Autodesk Inventor part; units mm, degrees
ref_plane "YZ Plane" through (0, 0, 0) normal (1, 0, 0) x (0, 1, 0)
ref_plane "XZ Plane" through (0, 0, 0) normal (0, 1, 0) x (-1, 0, 0)
ref_plane "XY Plane" through (0, 0, 0) normal (0, 0, 1) x (1, 0, 0)
sketch "Sketch1" plane through (0, 0, 0) normal (0, 1, 0) x (-1, 0, 0)
  line L0 (22.75, -10.36) -> (7.75, -10.36)
  line L1 (7.75, -10.36) -> (-0.1031, 0)
  circle A0 centre (4.34, -10.36) radius 1
  line L2 (22.75, 10.36) -> (7.75, 10.36)
  circle A1 centre (12.64, 0) radius 9.6 construction
  line L3 (22.75, 12.36) -> (22.75, -12.36)
  circle A2 centre (4.34, 10.36) radius 1
  line L4 (7.75, 10.36) -> (-0.1031, 0)
  line L5 (26.25, 19) -> (26.25, -19)
  line L6 (22.75, -12.36) -> (-22.75, -12.36)
  line L7 (22.75, 0) -> (-22.75, 0) construction
  line L8 (26.25, -19) -> (-28.75, -19)
  line L9 (26.25, -19) -> (-28.75, 19) construction
  line L10 (-28.75, -19) -> (26.25, 19) construction
  line L11 (-22.75, 12.36) -> (22.75, 12.36)
  line L12 (-28.75, 19) -> (26.25, 19)
  line L13 (-28.75, -19) -> (-28.75, 19)
  circle A3 centre (-16.36, 10.25) radius 1
  line L14 (-22.75, -12.36) -> (-22.75, 12.36)
  circle A4 centre (-16.36, -10.25) radius 1
  point P0 (0, 0)
  point P1 (-1.25, 0)
  point P2 (0, 0)
  point P3 (22.75, -10.36)
  dimension "d0" = 55
  dimension "d1" = 38
  dimension "d2" = 45.5
  dimension "d3" = 24.72
  dimension "d4" = 2
  dimension "d6" = 18.41
  dimension "d7" = 20.5
  dimension "d8" = 19.2
  dimension "d9" = 10.11
  dimension "d10" = 13
  dimension "d11" = 15
  dimension "d12" = 3.5
  dimension "d13" = 2
  dimension "d68" = 3.41
  dimension "d69" = 20.7
extrude "Extrusion1" add sketch "Sketch1" along normal mid plane 1 contours L3 L6 L14 L11 L2 L4 L1 L0 | L5 L8 L13 L12
extrude "Extrusion2" add sketch "Sketch1" along normal blind 35 contours L5 L8 L13 L12
fillet "Fillet1" radius 3 8 edges at (1.25, -0.5, -19) (28.75, -0.5, 0) (1.25, -0.5, 19) (-26.25, -0.5, 0) (28.75, 17.25, -19) (28.75, 17.25, 19) (-26.25, 17.25, 19) (-26.25, 17.25, -19)
sketch "Sketch6" plane through (28.75, 2.5, 16) normal (1, 0, 0) x (0, 0, -1)
  circle A0 centre (23, 14.75) radius 1.5
  line L0 (0, 32.5) -> (32, 32.5)
  line L1 (16, 32.5) -> (16, 0)
  line L2 (32, 0) -> (0, 0)
  line L3 (16, 39.5) -> (16, 7)
  circle A1 centre (23, 21.75) radius 1.5
  line L4 (16, 46.5) -> (16, 14)
  circle A2 centre (23, 28.75) radius 1.5
  line L5 (2, 32.5) -> (2, 0)
  circle A3 centre (9, 14.75) radius 1.5
  line L6 (2, 39.5) -> (2, 7)
  circle A4 centre (9, 21.75) radius 1.5
  line L7 (2, 46.5) -> (2, 14)
  circle A5 centre (9, 28.75) radius 1.5
  point P0 (16, -2.5)
  dimension "d50" = 3
  dimension "d54" = 7
  dimension "d57" = 14
  dimension "d70" = 3.75
hole "Hole2" at (28.75, 31.25, 7) at (28.75, 31.25, -7) at (28.75, 24.25, -7) at (28.75, 24.25, 7) at (28.75, 17.25, 7) at (28.75, 17.25, -7) direction (-1, 0, 0) diameter 4 depth 5 countersink diameter 4.2 countersink angle 90
sketch "Sketch7" plane through (0, 35, 0) normal (0, 1, 0) x (1, 0, 0)
  line L0 (-26.25, 16) -> (-26.25, -16)
  line L1 (-26.25, 0) -> (28.75, 0)
  line L2 (28.75, -16) -> (28.75, 16)
  line L3 (-23.25, -16) -> (25.75, -16)
  circle A0 centre (12.75, -16) radius 1.5
  circle A1 centre (12.75, 16) radius 1.5
  point P0 (0, 0)
  dimension "d71" = 3
  dimension "d72" = 16
hole "Hole3" at (12.75, 35, 16) at (12.75, 35, -16) direction (0, -1, 0) diameter 4 depth 7 countersink diameter 4.2 countersink angle 90
properties part number "basketback" material "PCTG 20%"
Part model, mm, in its own coordinate system. A direction names the side the tool comes from. Round coordinates to 2 decimals unless told otherwise and drop trailing zeros. Order: outer loops, then holes, each group sorted by start corner. A loop starts at its lowest first (then second) coordinate and runs counter-clockwise, first axis right, second up. Notation, with made-up numbers: M 60.25,25.25 L 97.25,25.25 A12 ccw 97.25,45.25 Z; hole C -34.5,15.25 d8. An arc over 180 degrees is marked long. Put each result on its own line as item: value. Start each with the question number.
1. Tool access for faces 4 (the face through (22.75, 18, 0)), 5 (the face through (-3.878, -0.007, 5.253)), 6 (the face through (23.75, 31, 7)), 7 (the face through (27.89, 18.98, -18.1)): list every direction of +Z, -Z, +X, -X, +Y, -Y with a clear straight run to the whole face (end or side of a thin tool).
2. Drop flat-ended pins along their axis: pin 1 (1.5 mm diameter, centred on x = -20, z = -9.5, fed in from -Y); pin 2 (2.5 mm diameter, centred on x = 16.36, z = 10.25, fed in from +Y); pin 3 (1.1 mm diameter, centred on x = -11.5, y = 0, fed in from +Z); pin 4 (1.2 mm diameter, centred on y = 17, z = -6, fed in from +X). Give the stop position or say it passes through.
3. Two-plate mould, pull along X, no slides. Class faces 1 (the face through (-3.878, -0.007, -5.253)), 2 (the face through (-25.39, 18.98, 18.1)), 3 (the face through (27.85, 0.36, 0.22)): +X half, -X half, draft (parallel to the pull), parting line (faces both ways), or undercut.
4. Slice it at B-B on y = 24.25. List the corners of the cut face in (x, z), then the cut area to 3 significant figures.
5. Drill centre lines: probe 1 along Y at (x, z) = (25.55, 7); probe 2 along Z at (x, y) = (3.5, 18); probe 3 along X at (y, z) = (22.5, 2.5). Where is each one in solid material? Low to high. Write a range as [from, to].
6. Slice it at A-A on x = -12.5. List the corners of the cut face in (y, z), then the cut area to 3 significant figures.
7. Slice it at C-C on z = -3.5. List the corners of the cut face in (x, y), then the cut area to 3 significant figures.
8. Slice it at D-D on y = 31.25. List the corners of the cut face in (x, z).
Findings:
1. face 4: +Y
1. face 5: +Y, -Y
1. face 6: +X
1. face 7: -Z, +X, +Y, -Y
2. pin 1: through
2. pin 2: y = 0.5
2. pin 3: z = 18.28
2. pin 4: x = 23.75
3. face 1: undercut
3. face 2: -X half
3. face 3: +X half
4. outline: M -26.25,-16 A3 ccw -23.25,-19 L 25.75,-19 A3 ccw 28.75,-16 L 28.75,-9.1 L 28.65,-9 L 23.75,-9 L 23.75,-5 L 28.65,-5 L 28.75,-4.9 L 28.75,4.9 L 28.65,5 L 23.75,5 L 23.75,9 L 28.65,9 L 28.75,9.1 L 28.75,16 A3 ccw 25.75,19 L -23.25,19 A3 ccw -26.25,16 Z; hole M -22.75,-12.36 L 22.75,-12.36 L 22.75,12.36 L -22.75,12.36 Z
4. area: 917 mm2
5. probe 1: [-0.5, 15.25], [19.25, 22.25], [26.25, 29.25], [33.25, 35]
5. probe 2: [-19, -12.36], [12.36, 19]
5. probe 3: [-26.25, -22.75], [22.75, 28.75]
6. outline: M -0.5,-16 A3 ccw 2.5,-19 L 35,-19 L 35,-12.36 L 0.5,-12.36 L 0.5,-10.36 L -0.5,-10.36 Z; M -0.5,10.36 L 0.5,10.36 L 0.5,12.36 L 35,12.36 L 35,19 L 2.5,19 A3 ccw -0.5,16 Z
6. area: 472 mm2
7. outline: M -26.25,2.5 A3 ccw -23.25,-0.5 L -22.75,-0.5 L -22.75,35 L -26.25,35 Z; M -2.55,-0.5 L 25.75,-0.5 A3 ccw 28.75,2.5 L 28.75,35 L 22.75,35 L 22.75,0.5 L -2.55,0.5 Z
7. area: 359 mm2
8. outline: M -26.25,-16 A3 ccw -23.25,-19 L 25.75,-19 A3 ccw 28.75,-16 L 28.75,-9.1 L 28.65,-9 L 23.75,-9 L 23.75,-5 L 28.65,-5 L 28.75,-4.9 L 28.75,4.9 L 28.65,5 L 23.75,5 L 23.75,9 L 28.65,9 L 28.75,9.1 L 28.75,16 A3 ccw 25.75,19 L -23.25,19 A3 ccw -26.25,16 Z; hole M -22.75,-12.36 L 22.75,-12.36 L 22.75,12.36 L -22.75,12.36 Z; hole C 12.75,-16 d4; hole C 12.75,16 d4
